from build123d import *

# Parameters (mm, degrees)
SKETCH004_W              = 18
SKETCH004_H              = 169.6125627158
PAD003_DEPTH             = 5
SKETCH005_W              = 18
SKETCH005_H              = 56.5375209053
PAD004_DEPTH             = 10
PAD005_DEPTH             = 18
SKETCH007_W              = 93.8062813579
SKETCH007_H              = 10
POCKET_DEPTH             = 2.5
SKETCH008_W              = 93.8062813579
SKETCH008_H              = 10
POCKET001_DEPTH          = 2.5
CLONE024_PITCH_ANGLE     = 90
CLONE024_PLACEMENT_ANGLE = -90


with BuildPart() as part:
    # Sketch004 → Pad003 (new body)
    with BuildSketch(Plane.XY):
        with Locations((0, -97.1937186421)):
            Rectangle(SKETCH004_W, SKETCH004_H)
    extrude(amount=PAD003_DEPTH)

    # Sketch005 (on Face5 of Pad003) → Pad004 (join)
    with BuildSketch(Plane(origin=(0, 0, 0), x_dir=(1, 0, 0), z_dir=(0, 0, -1))):
        with Locations((0, 97.1937186421)):
            Rectangle(SKETCH005_W, SKETCH005_H)
    extrude(amount=PAD004_DEPTH)

    # Sketch006 (on Face9 of Pad004) → Pad005 (join)
    with BuildSketch(Plane.YZ.offset(9)):
        Polygon((-12.3874372842, 0), (-68.9249581895, 0), (-68.9249581895, -10), (-125.4624790947, -10), (-125.4624790947, 0), (-182, 0), (-182, 5), (-200, 5), (-200, 375), (-182, 375), (-182, 380), (-125.4624790947, 380), (-125.4624790947, 390), (-68.9249581895, 390), (-68.9249581895, 380), (-12.3874372842, 380), (-12.3874372842, 375), (-12.3874372842, 258.3333333333), (-106.1937186421, 258.3333333333), (-106.1937186421, 248.3333333333), (-12.3874372842, 248.3333333333), (-12.3874372842, 131.6666666667), (-106.1937186421, 131.6666666667), (-106.1937186421, 121.6666666667), (-12.3874372842, 121.6666666667), (-12.3874372842, 5), align=None)
    extrude(amount=-PAD005_DEPTH)

    # Sketch007 (on Face11 of Pad005) → Pocket (cut)
    with BuildSketch(Plane.YZ.offset(9)):
        with Locations((-153.0968593211, 253.3333333333)):
            Rectangle(SKETCH007_W, SKETCH007_H)
        with Locations((-153.0968593211, 126.6666666667)):
            Rectangle(SKETCH007_W, SKETCH007_H)
    extrude(amount=-POCKET_DEPTH, mode=Mode.SUBTRACT)

    # Sketch008 (on Face9 of Pocket) → Pocket001 (cut)
    with BuildSketch(Plane(origin=(-9, 0, 0), x_dir=(0, -1, 0), z_dir=(-1, 0, 0))):
        with Locations((153.0968593211, 126.6666666667)):
            Rectangle(SKETCH008_W, SKETCH008_H)
        with Locations((153.0968593211, 253.3333333333)):
            Rectangle(SKETCH008_W, SKETCH008_H)
    extrude(amount=-POCKET001_DEPTH, mode=Mode.SUBTRACT)


with BuildPart() as part_1:
    # Body004 placement: moved
    add(part.part.moved(Location((0, 0, 13))))


with BuildPart() as part_2:
    # Clone024 pitch: moved
    add(part_1.part.rotate(Axis((0, 0, 0), (0, 1, 0)), CLONE024_PITCH_ANGLE))


with BuildPart() as part_3:
    # Clone024 placement: moved
    add(part_2.part.moved(Location((0, 203, 9))).rotate(Axis((0, 203, 9), (0, 0, 1)), CLONE024_PLACEMENT_ANGLE))


solid = part_3.part
Input: part model. Units: mm. Frame: model coordinates. A direction names the side the tool comes from. Round coordinates to 2 decimals unless told otherwise and drop trailing zeros. Loops run counter-clockwise (first coordinate to the right, second up) from the corner with the lowest first, then second, coordinate; pieces in that order, holes last. Notation, with made-up numbers: M -25.5,-2 L -4.5,-2 A10 cw -4.5,4 Z; hole C 28.25,82.5 d8. An arc over 180 degrees is marked long. Answer as CSV lines item,"result". Start each with the question number.
(1) Reachability of faces 5 (the flat face through (-153, 190, 9)), 6 (the flat face through (-106.194, 63, 9)), 7 (the flat face through (-125.462, -195, 9)), 8 (the flat face through (-41, -190, 9)) from +Z, -Z, +X, -X, +Y, -Y: full face, straight path, thin tool, end or side. Return the list, or none.
(2) Section A-A, the plane x = -97.5. Output: boundary loops of the cut face in (y, z).
(3) Draft query along Y for faces 1 (the flat face through (-154, 63, 2.5)), 2 (the flat face through (-40, 190, 9)), 3 (the flat face through (-108, 1, 18)), 4 (the flat face through (-191, -185, 9)). Return one class per face: released by +Y, released by -Y, zero draft, split by the parting line, or undercut.
(4) Section D-D, the plane x = -51.5. Output: boundary loops of the cut face in (y, z).
(5) Section C-C, the plane z = 5.5. Output: boundary loops of the cut face in (x, y).
(6) First-contact query: pin 1 (3 mm diameter, centred on x = -138.5, y = -64.5, fed in from -Z); pin 2 (8 mm diameter, centred on y = 196.5, z = 7, fed in from +X); pin 3 (3 mm diameter, centred on x = -36, z = 4, fed in from -Y). Flat tips, straight axial feed; report the tip coordinate or a pass-through.
(7) Line query: line 1 (Y direction, x = -57, z = 3.25); line 2 (Y direction, x = -94, z = 3.5); line 3 (Y direction, x = -151, z = 13.5). Output: solid intervals per line, ascending. Write a range as [from, to].
(8) Section B-B, the plane x = -153. Output: boundary loops of the cut face in (y, z), plus the area to 3 significant figures.
Values found:
1,face 5,"+Z, -Z, -X, +Y"
1,face 6,"+Z, -Z, +X"
1,face 7,"+Z, -Z, -X, -Y"
1,face 8,"+Z, -Z, +X, -Y"
2,outline,"M -200,0 L -68.33,0 L -68.33,18 L -200,18 Z; M -58.33,0 L 58.33,0 L 58.33,18 L -58.33,18 Z; M 68.33,0 L 200,0 L 200,18 L 68.33,18 Z"
3,face 1,"undercut"
3,face 2,"released by +Y"
3,face 3,"zero draft"
3,face 4,"released by -Y"
4,outline,"M -190,0 L -68.33,0 L -68.33,18 L -190,18 Z; M -58.33,0 L 58.33,0 L 58.33,18 L -58.33,18 Z; M 68.33,0 L 190,0 L 190,18 L 68.33,18 Z"
5,outline,"M -200,-185 L -182,-185 L -182,-190 L -125.46,-190 L -125.46,-200 L -68.92,-200 L -68.92,-190 L -12.39,-190 L -12.39,-68.33 L -106.19,-68.33 L -106.19,-58.33 L -12.39,-58.33 L -12.39,58.33 L -106.19,58.33 L -106.19,68.33 L -12.39,68.33 L -12.39,190 L -68.92,190 L -68.92,200 L -125.46,200 L -125.46,190 L -182,190 L -182,185 L -200,185 Z"
6,pin 1,"stops at z = 2.5"
6,pin 2,"stops at x = -68.92"
6,pin 3,"stops at y = -190"
7,line 1,"y = [-190, -68.33], [-58.33, 58.33], [68.33, 190]"
7,line 2,"y = [-200, -68.33], [-58.33, 58.33], [68.33, 200]"
7,line 3,"y = [-190, 190]"
8,outline,"M -190,0 L -68.33,0 L -68.33,2.5 L -58.33,2.5 L -58.33,0 L 58.33,0 L 58.33,2.5 L 68.33,2.5 L 68.33,0 L 190,0 L 190,18 L 68.33,18 L 68.33,15.5 L 58.33,15.5 L 58.33,18 L -58.33,18 L -58.33,15.5 L -68.33,15.5 L -68.33,18 L -190,18 Z"
8,area,"6,740 mm²"
